```python
from build123d import *

# Parameters (mm, degrees)
EXTRUDE_2_DEPTH             = 1
F_3_0MM_1_D                 = 3
F_3_0MM_1_DEPTH             = 4
F_3_0MM_1_TIP               = 0.901290929
F_3_0MM_1_ON_FACE_2_D       = 3
F_3_0MM_1_ON_FACE_2_DEPTH   = 4
F_3_0MM_1_ON_FACE_2_TIP     = 0.901290929
PATTERN_LINEAR_1_COUNT      = 2
PATTERN_LINEAR_1_PITCH      = 98
PATTERN_LINEAR_1_COUNT_DIR2 = 2
PATTERN_LINEAR_1_PITCH_DIR2 = 44
SKETCH_16_W                 = 4
SKETCH_16_H                 = 15
EXTRUDE_3_DEPTH             = 13
CUT_EXTRUDE_1_REACH         = 107.413
SKETCH_17_W                 = 11
SKETCH_17_H                 = 11
SKETCH_18_W                 = 18
SKETCH_18_H                 = 14.2
SKETCH_18_W_2               = 16
SKETCH_18_H_2               = 12.2
EXTRUDE_4_DEPTH             = 3


with BuildPart() as part:
    # 草圖10 → 填料-伸長2 (new body)
    with BuildSketch(Plane(origin=(0, 0, 0), x_dir=(1, 0, 0), z_dir=(0, 1, 0))):
        with BuildLine():
            Line((56.568542495, 34), (-56.568542495, 34))
            ThreePointArc((-56.568542495, 34), (-61.540159626, 23.849711805), (-64.707032075, 13))
            Line((-64.707032075, 13), (-56.707032075, 13))
            Line((-56.707032075, 13), (-56.707032075, -12.973279994))
            Line((-56.707032075, -12.973279994), (-64.707032075, -13))
            ThreePointArc((-64.707032075, -13), (-61.540159626, -23.849711805), (-56.568542495, -34))
            Line((-56.568542495, -34), (56.568542495, -34))
            ThreePointArc((56.568542495, -34), (61.619473981, -23.644035746), (64.792427449, -12.567471713))
            Line((64.792427449, -12.567471713), (56.707032075, -12.594476939))
            Line((56.707032075, -12.594476939), (56.707032075, 13))
            Line((56.707032075, 13), (64.707032075, 13))
            ThreePointArc((64.707032075, 13), (61.540159626, 23.849711805), (56.568542495, 34))
        make_face()
    extrude(amount=EXTRUDE_2_DEPTH)

    # Ø3.0mm 定位孔1
    with Locations(Plane(origin=(30, 1, 30), x_dir=(0, 0, 1), z_dir=(0, 1, 0))):
        with Locations((0, 0), (-60, -60), (0, -60), (-60, 0)):
            Hole(F_3_0MM_1_D / 2, depth=F_3_0MM_1_DEPTH)
            with Locations((0, 0, -(F_3_0MM_1_DEPTH + F_3_0MM_1_TIP / 2))):  # 118° drill point
                Cone(0, F_3_0MM_1_D / 2, F_3_0MM_1_TIP, mode=Mode.SUBTRACT)

    # Ø3.0mm 定位孔1 on face 2
    with Locations(Plane(origin=(-30, 0, -30), x_dir=(0, 0, -1), z_dir=(0, -1, 0))):
        with Locations((0, 0)):
            Hole(F_3_0MM_1_ON_FACE_2_D / 2, depth=F_3_0MM_1_ON_FACE_2_DEPTH)
            with Locations((0, 0, -(F_3_0MM_1_ON_FACE_2_DEPTH + F_3_0MM_1_ON_FACE_2_TIP / 2))):  # 118° drill point
                Cone(0, F_3_0MM_1_ON_FACE_2_D / 2, F_3_0MM_1_ON_FACE_2_TIP, mode=Mode.SUBTRACT)

    # 草圖14 → Ø3.0mm 定位孔2 (revolve, cut)
    with BuildSketch(Plane(origin=(-49, 1, -22), x_dir=(0, 0, 1), z_dir=(1, 0, 0))):
        Polygon((0, 0), (0, 4.901290929), (1.5, 4), (1.5, 0), align=None)
    f_3_0mm_2 = revolve(axis=Axis((-49, 7.35, -22), (0, -1, 0)), mode=Mode.SUBTRACT)

    # 直線複製排列1: 3.0mm _2 2 × 2
    with Locations(*[(i * PATTERN_LINEAR_1_PITCH, 0, j * PATTERN_LINEAR_1_PITCH_DIR2) for i in range(PATTERN_LINEAR_1_COUNT) for j in range(PATTERN_LINEAR_1_COUNT_DIR2) if (i, j) != (0, 0)]):
        add(f_3_0mm_2, mode=Mode.SUBTRACT)

    # 草圖16 → 填料-伸長3 (add)
    with BuildSketch(Plane(origin=(0, 1, 0), x_dir=(1, 0, 0), z_dir=(0, 1, 0))):
        with Locations((-32, 10)):
            Rectangle(SKETCH_16_W, SKETCH_16_H)
        with Locations((32, 10)):
            Rectangle(SKETCH_16_W, SKETCH_16_H)
        with Locations((32, -10)):
            Rectangle(SKETCH_16_W, SKETCH_16_H)
        with Locations((-32, -10)):
            Rectangle(SKETCH_16_W, SKETCH_16_H)
    extrude(amount=EXTRUDE_3_DEPTH)

    # 除料-伸長1: up to this face of the body (flat: up to its plane)
    cut_extrude_1_end = Plane(part.part.faces().sort_by_distance((34, 7.5, -10))[0])
    # 草圖17 → 除料-伸長1 (cut, up to the picked face)
    with BuildSketch(Plane.ZY.offset(34), mode=Mode.PRIVATE) as cut_extrude_1_sk1:
        with Locations((-10, 6.5)):
            Rectangle(SKETCH_17_W, SKETCH_17_H)
    cut_extrude_1_tool1 = split(extrude(cut_extrude_1_sk1.sketch, amount=-CUT_EXTRUDE_1_REACH, mode=Mode.PRIVATE), bisect_by=cut_extrude_1_end, keep=Keep.BOTH, mode=Mode.PRIVATE)
    # 草圖17 → 除料-伸長1 (cut, up to the picked face)
    with BuildSketch(Plane.ZY.offset(34), mode=Mode.PRIVATE) as cut_extrude_1_sk2:
        with Locations((10, 6.5)):
            Rectangle(SKETCH_17_W, SKETCH_17_H)
    cut_extrude_1_tool2 = split(extrude(cut_extrude_1_sk2.sketch, amount=-CUT_EXTRUDE_1_REACH, mode=Mode.PRIVATE), bisect_by=cut_extrude_1_end, keep=Keep.BOTH, mode=Mode.PRIVATE)
    add(cut_extrude_1_tool1.solids().sort_by(Axis((-34, 6.5, -10), (1, 0, 0)))[0], mode=Mode.SUBTRACT)
    add(cut_extrude_1_tool2.solids().sort_by(Axis((-34, 6.5, 10), (1, 0, 0)))[0], mode=Mode.SUBTRACT)

    # 草圖18 → 填料-伸長4 (add)
    with BuildSketch(Plane(origin=(0, 1, 0), x_dir=(1, 0, 0), z_dir=(0, 1, 0))):
        with Locations((-8.938019144, 23.21731374)):
            Rectangle(SKETCH_18_W, SKETCH_18_H)
        with Locations((-8.938019144, 23.21731374)):
            Rectangle(SKETCH_18_W_2, SKETCH_18_H_2, mode=Mode.SUBTRACT)
    extrude(amount=EXTRUDE_4_DEPTH)


solid = part.part
```
For this review, take the finished solid that the model builds, in its own axes (mm). A direction names the side the tool comes from. Round coordinates to 2 decimals unless told otherwise and drop trailing zeros. Write each loop counter-clockwise with the first axis right and the second up, starting at its lowest first coordinate (ties: lowest second). Pieces come first, ordered by that corner, then holes. Notation, with made-up numbers: (-7, 41.5) - (33, 41.5) arc R27 cw to (33, 66.5) - close; hole circle Ø8 at (-11.5, 86.5). An arc over 180 degrees is marked (long way). Answer as CSV lines item,"result". Start each with the question number.
(1) For line 1 (Z direction, x = 49, y = 0.6); line 2 (X direction, y = 2, z = -21); line 3 (X direction, y = 13.25, z = -7), list the stretches that pass through material, from the lowest coordinate up.
(2) Add section B-B, the plane y = 9.5. State how many separate pieces and enclosed holes the cut face has, plus the area to 3 significant figures.
(3) Mouldability with a two-part tool opening along X and no side actions: class faces 1 (the flat face through (32, 7, 2.5)), 2 (the cylindrical face through (50.464, 0.507, -22.325)), 3 (the flat face through (-34, 12.3, -10)) as +X half, -X half, draft (parallel to the pull), parting line (faces both ways), or undercut.
(4) Add section A-A, the plane x = -49. State the section outline as (y, z) points.
(5) Add section D-D, the plane x = -12.5. State the section outline as (y, z) points, plus the area to 3 significant figures.
(6) For pin 1 (3 mm diameter, centred on x = -32.5, y = 5, fed in from -Z); pin 2 (2.5 mm diameter, centred on y = 2, z = -21, fed in from +X); pin 3 (4.5 mm diameter, centred on x = -31, y = 7, fed in from +Z), all flat-tipped, find the tip position at first contact; note any pin that passes through.
(7) Add section C-C, the plane z = -9.5. State the section outline as (x, y) points.
(8) Machinability: for faces 4 (the flat face through (32, 6, -4.5)), 5 (the flat face through (-9, 2, -16.117)), 6 (the flat face through (-32, 7, 17.5)), which of the approach directions +Z, -Z, +X, -X, +Y, -Y give a long, thin tool a straight path to every point of the face, cutting with its end or side? Answer none if there is none.
From the geometry:
1,line 1,"z = -34 to -23.5, -20.5 to 20.5, 23.5 to 34"
1,line 2,"x = -17.94 to -16.94, -0.94 to 0.06"
1,line 3,"x = -34 to -30, 30 to 34"
2,separate pieces,"8"
2,enclosed holes,"0"
2,area,"64.0 mm²"
3,face 1,"draft"
3,face 2,"undercut"
3,face 3,"-X half"
4,outline,"(0, -34) - (1, -34) - (1, -23.5) - (0, -23.5) - close; (0, -20.5) - (1, -20.5) - (1, 20.5) - (0, 20.5) - close; (0, 23.5) - (1, 23.5) - (1, 34) - (0, 34) - close"
5,outline,"(0, -34) - (1, -34) - (1, -30.32) - (4, -30.32) - (4, -29.32) - (1, -29.32) - (1, -17.12) - (4, -17.12) - (4, -16.12) - (1, -16.12) - (1, 34) - (0, 34) - close"
5,area,"74.0 mm²"
6,pin 1,"stops at z = -17.5"
6,pin 2,"stops at x = 62.82"
6,pin 3,"stops at z = 17.5"
7,outline,"(-56.71, 0) - (56.71, 0) - (56.71, 1) - (-56.71, 1) - close; (-34, 12) - (-30, 12) - (-30, 14) - (-34, 14) - close; (30, 12) - (34, 12) - (34, 14) - (30, 14) - close"
8,face 4,"+X, -X"
8,face 5,"+Z, +Y"
8,face 6,"+Z, +X, -X, +Y"
